Part print with two shaded views. Sizes in mm from the minimum x, y, z corner. Round coordinates to 2 decimals unless told otherwise and drop trailing zeros. Write each loop counter-clockwise with the first axis right and the second up, starting at its lowest first coordinate (ties: lowest second). Pieces come first, ordered by that corner, then holes. Notation, with made-up numbers: (-38.75, 19.25) -> (17.25, 19.25) arc R37 ccw to (17.25, 57.25) -> close; hole circle Ø4 at (-24.5, -34.75). An arc over 180 degrees is marked (long way). Answer in a Markdown table with one row per item.
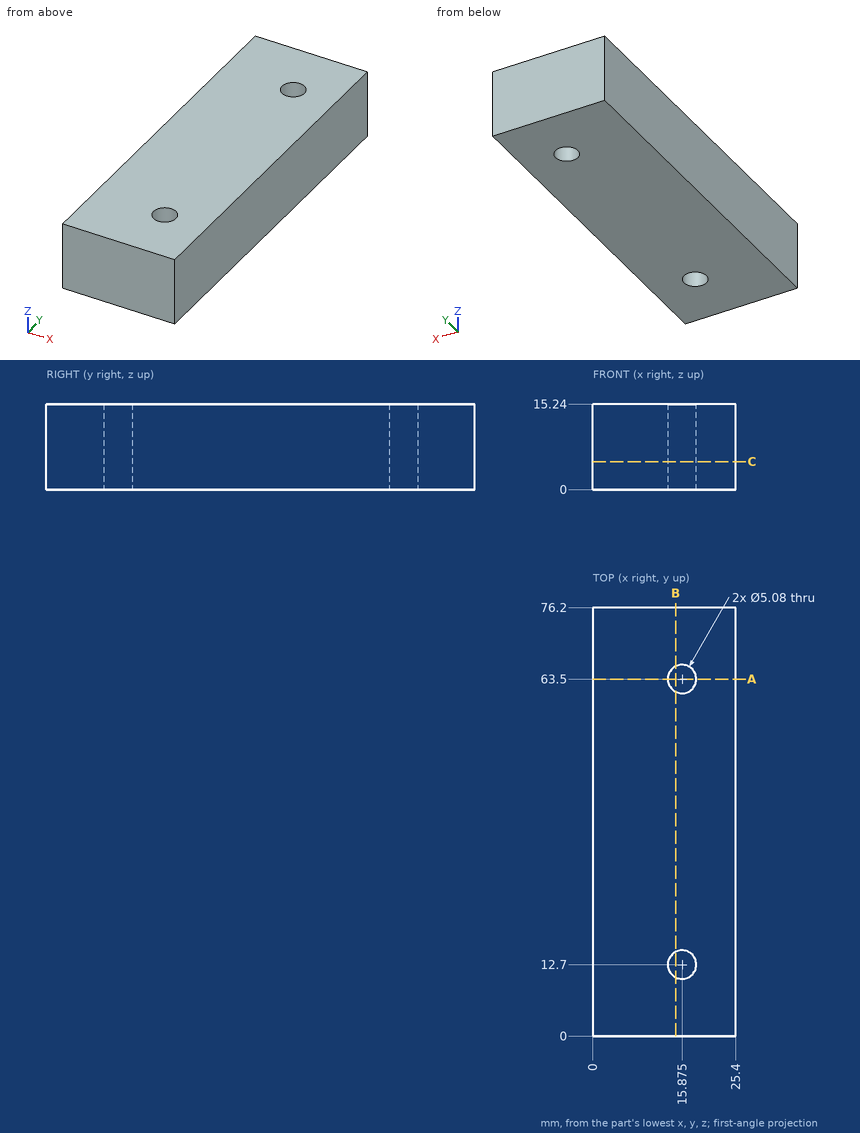
Q1. Saw through at C-C on z = 5. Write the cut outline in (x, y) (3 decimals).
A:
| item | result |
|---|---|
| outline | (0, 0) -> (25.4, 0) -> (25.4, 76.2) -> (0, 76.2) -> close; hole circle Ø5.08 at (15.875, 12.7); hole circle Ø5.08 at (15.875, 63.5) |
Q2. Saw through at A-A on y = 63.5. Write the cut outline in (x, z) (3 decimals).
A:
| item | result |
|---|---|
| outline | (0, 0) -> (13.335, 0) -> (13.335, 15.24) -> (0, 15.24) -> close; (18.415, 0) -> (25.4, 0) -> (25.4, 15.24) -> (18.415, 15.24) -> close |
Q3. Saw through at B-B on x = 14.75. Write the cut outline in (y, z), plus the area to 3 significant figures.
A:
| item | result |
|---|---|
| outline | (0, 0) -> (10.42, 0) -> (10.42, 15.24) -> (0, 15.24) -> close; (14.98, 0) -> (61.22, 0) -> (61.22, 15.24) -> (14.98, 15.24) -> close; (65.78, 0) -> (76.2, 0) -> (76.2, 15.24) -> (65.78, 15.24) -> close |
| area | 1,020 mm² |
Q4. Wall check: line 1 (Y direction, x = 14.5, z = 13); line 2 (Y direction, x = 16.75, z = 12.75); line 3 (X direction, y = 62, z = 4.25). Give the ranges that are in metal, low to high. Write a range as [from, to].
A:
| item | result |
|---|---|
| line 1 | [0, 10.56], [14.84, 61.36], [65.64, 76.2] |
| line 2 | [0, 10.32], [15.08, 61.12], [65.88, 76.2] |
| line 3 | [0, 13.83], [17.92, 25.4] |
